The model under review builds one solid part; all positions refer to its coordinate system, in mm. A direction names the side the tool comes from. Coordinates: 2 decimals unless noted, no trailing zeros. Order: outer loops, then holes, each group sorted by start corner. A loop starts at its lowest first (then second) coordinate and runs counter-clockwise, first axis right, second up. Notation, with made-up numbers: (22.25, 48) -> (44.25, 48) arc R33 ccw to (44.25, 86) -> close; hole circle Ø5 at (-7.75, 83). An arc over 180 degrees is marked (long way). Use one line per item in the form item = value.
from build123d import *

# Parameters (mm, degrees)
BOSS_EXTRUDE1_DEPTH = 32
SKETCH2_W           = 35.6
SKETCH2_H           = 29.2
BOSS_EXTRUDE2_DEPTH = 3
BOSS_EXTRUDE3_DEPTH = 3
SKETCH4_R           = 1.5
CUT_EXTRUDE1_DEPTH  = 4


with BuildPart() as part:
    # Sketch1 → Boss-Extrude1 (new body)
    with BuildSketch(Plane.XY):
        with BuildLine():
            Line((0, 0), (-19.7, 0))
            Line((-19.7, 0), (-19.7, 29.2))
            Line((-19.7, 29.2), (-20, 29.2))
            Line((-20, 29.2), (-55, 29.2))
            Line((-55, 29.2), (-55.3, 29.2))
            Line((-55.3, 29.2), (-55.3, 0))
            Line((-55.3, 0), (-75, 0))
            ThreePointArc((-75, 0), (-76.5, 1.5), (-75, 3))
            Line((-75, 3), (-58, 3))
            Line((-58, 3), (-58, 30.2))
            Line((-58, 30.2), (-58, 32.2))
            Line((-58, 32.2), (-17, 32.2))
            Line((-17, 32.2), (-17, 30.2))
            Line((-17, 30.2), (-17, 3))
            Line((-17, 3), (0, 3))
            ThreePointArc((0, 3), (1.5, 1.5), (0, 0))
        make_face()
    extrude(amount=BOSS_EXTRUDE1_DEPTH)

    # Sketch2 → Boss-Extrude2 (add)
    with BuildSketch(Plane(origin=(0, 0, 0), x_dir=(-1, 0, 0), z_dir=(0, 0, -1))):
        with Locations((37.5, 14.6)):
            Rectangle(SKETCH2_W, SKETCH2_H)
        with BuildLine():
            Line((17, 3), (0, 3))
            ThreePointArc((0, 3), (-1.5, 1.5), (0, 0))
            Line((0, 0), (19.7, 0))
            Line((19.7, 0), (19.7, 29.2))
            Line((19.7, 29.2), (55.3, 29.2))
            Line((55.3, 29.2), (55.3, 0))
            Line((55.3, 0), (75, 0))
            ThreePointArc((75, 0), (76.5, 1.5), (75, 3))
            Line((75, 3), (58, 3))
            Line((58, 3), (58, 32.2))
            Line((58, 32.2), (17, 32.2))
            Line((17, 32.2), (17, 3))
        make_face()
    extrude(amount=BOSS_EXTRUDE2_DEPTH)

    # Sketch3 → Boss-Extrude3 (add)
    with BuildSketch(Plane.XY.offset(32)):
        with BuildLine():
            Line((-20, 0), (-23, 0))
            Line((-23, 0), (-23, 3))
            Line((-23, 3), (-20, 3))
            Line((-20, 3), (0, 3))
            ThreePointArc((0, 3), (1.5, 1.5), (0, 0))
            Line((0, 0), (-20, 0))
        make_face()
        with BuildLine():
            Line((-55, 0), (-75, 0))
            ThreePointArc((-75, 0), (-76.5, 1.5), (-75, 3))
            Line((-75, 3), (-55, 3))
            Line((-55, 3), (-52, 3))
            Line((-52, 3), (-52, 0))
            Line((-52, 0), (-55, 0))
        make_face()
    extrude(amount=BOSS_EXTRUDE3_DEPTH)

    # Sketch4 → Cut-Extrude1 (cut)
    with BuildSketch(Plane.XZ):
        with Locations((-65, 16)):
            Circle(SKETCH4_R)
        with Locations((-10, 16)):
            Circle(SKETCH4_R)
    extrude(amount=-CUT_EXTRUDE1_DEPTH, mode=Mode.SUBTRACT)


solid = part.part
Item 1: Draft analysis for pull direction X (two halves, no side actions). For faces 1 (the face through (-37, 30, 32)), 2 (the face through (-52, 2, 33)), 3 (the face through (1.5, 1.5, 15.7)), 4 (the face through (-55.3, 15, 16)), state which applies: released by +X, released by -X, zero draft, split by the parting line, or undercut.
Results found:
face_1 = zero draft
face_2 = undercut
face_3 = released by +X
face_4 = undercut
Item 2: We need section B-B (x = -65). Write out the cut boundary in (y, z).
Results found:
outline = (0, -3) -> (3, -3) -> (3, 14.5) -> (0, 14.5) -> close; (0, 17.5) -> (3, 17.5) -> (3, 35) -> (0, 35) -> close
Item 3: Tool access review of faces 5 (the face through (-37, 29.2, 16)), 6 (the face through (-58, 17, 15)), 7 (the face through (-23, 1, 33)), 8 (the face through (-76.5, 1.5, 16.3)), 9 (the face through (-21, 2, 32)): name each direction out of +Z, -Z, +X, -X, +Y, -Y from which nothing blocks a thin tool from reaching the whole face with its end or side.
Results found:
face_5 = +Z, -Y
face_6 = +Z, -Z, -X, +Y
face_7 = +Z, +Y, -Y
face_8 = +Z, -Z, -X
face_9 = -Y
Item 4: We need section C-C (y = 1.5). Write out the cut boundary in (x, z).
Results found:
outline = (-76.5, -3) -> (1.5, -3) -> (1.5, 35) -> (-23, 35) -> (-23, 32) -> (-19.7, 32) -> (-19.7, 0) -> (-55.3, 0) -> (-55.3, 32) -> (-52, 32) -> (-52, 35) -> (-76.5, 35) -> close; hole circle Ø3 at (-65, 16); hole circle Ø3 at (-10, 16)
Item 5: Clearance check with flat-ended pins moving along their axes: pin 1 (5 mm diameter, centred on x = -37, y = 11, fed in from +Z); pin 2 (10 mm diameter, centred on x = -50, z = 10, fed in from -Y); pin 3 (7 mm diameter, centred on x = -8, z = 8.5, fed in from +Y); pin 4 (2.5 mm diameter, centred on x = -10, z = 16, fed in from -Y) (3 decimals). State where each tip first meets the part, or that it passes through.
Results found:
pin_1 = 0
pin_2 = 29.2
pin_3 = 3
pin_4 = through
Item 6: We need section D-D (z = 27.5). Write out the cut boundary in (x, y), plus the area to 3 significant figures.
Results found:
outline = (-75, 0) -> (-55.3, 0) -> (-55.3, 29.2) -> (-19.7, 29.2) -> (-19.7, 0) -> (0, 0) arc R1.5 ccw to (0, 3) -> (-17, 3) -> (-17, 32.2) -> (-58, 32.2) -> (-58, 3) -> (-75, 3) arc R1.5 ccw to start
area = 390 mm²
Item 7: To check wall thickness, follow L1, parallel to X at y = 28, z = 20.5; L2, parallel to Z at x = -10, y = 1; L3, parallel to Y at x = -3, z = 4. State the ranges of each line that lie inside material, in increasing order. Write a range as from..to.
Results found:
L1 = -58..-55.3, -19.7..-17
L2 = -3..14.5, 17.5..35
L3 = 0..3
Item 8: We need section A-A (z = 16). Write out the cut boundary in (x, y), plus the area to 3 significant figures.
Results found:
outline = (-75, 0) -> (-66.5, 0) -> (-66.5, 3) -> (-75, 3) arc R1.5 ccw to start; (-63.5, 0) -> (-55.3, 0) -> (-55.3, 29.2) -> (-19.7, 29.2) -> (-19.7, 0) -> (-11.5, 0) -> (-11.5, 3) -> (-17, 3) -> (-17, 32.2) -> (-58, 32.2) -> (-58, 3) -> (-63.5, 3) -> close; (-8.5, 0) -> (0, 0) arc R1.5 ccw to (0, 3) -> (-8.5, 3) -> close
area = 372 mm²
